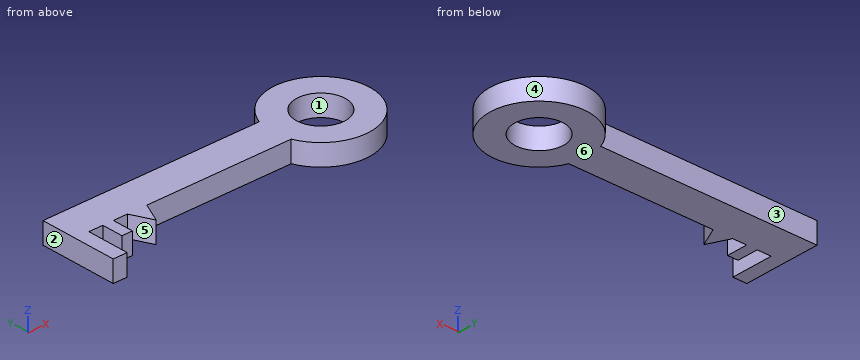
from build123d import *

# Parameters (mm, degrees)
F0_W     = 7.5505197141
F0_H     = 15
F0_W_2   = 10
F0_H_2   = 30
F0_R     = 17.5
F1_DEPTH = 15


# Not quite as in the source:
# - a feature of the source that left no trace in its solid (it failed there, or was rolled back) is left out


with BuildPart() as f1:
    # F0 (on Top) → F1 (new body)
    with BuildSketch(Plane.XY):
        Polygon((63.855322471, 51.9168977576), (-91.144677529, 51.9168977576), (-91.144677529, 26.9168977576), (-81.144677529, 26.9168977576), (-71.144677529, 26.9168977576), (-63.594157815, 26.9168977576), (-53.594157815, 26.9168977576), (-46.594157815, 26.9168977576), (-39.594157815, 26.9168977576), (63.855322471, 26.9168977576), align=None)
        Polygon((-46.594157815, 11.9168977576), (-39.594157815, 26.9168977576), (-46.594157815, 26.9168977576), (-53.594157815, 26.9168977576), align=None)
        with Locations((-67.369417672, 19.4168977576)):
            Rectangle(F0_W, F0_H)
        with Locations((-86.144677529, 11.9168977576)):
            Rectangle(F0_W_2, F0_H_2)
        with BuildLine():
            ThreePointArc((63.855322471, 26.9168977576), (131.5470645475, 39.4168977576), (63.855322471, 51.9168977576))
            Line((63.855322471, 51.9168977576), (63.855322471, 26.9168977576))
        make_face()
        with Locations((96.5470645475, 39.4168977576)):
            Circle(F0_R, mode=Mode.SUBTRACT)
    extrude(amount=F1_DEPTH)


solid = f1.part
Verification items for the finished model (mm, model axes). Face numbers are marked on the shaded views. A direction names the side the tool comes from. Give positions to 0.01 mm unless a question says otherwise; leave off trailing zeros. Order: outer loops, then holes, each group sorted by start corner. A loop starts at its lowest first (then second) coordinate and runs counter-clockwise, first axis right, second up. Notation, with made-up numbers: M 15,31 L 57,31 A28 ccw 57,56 Z; hole C 11.5,80 d10. An arc over 180 degrees is marked long. Use one line per item in the form item = value. Start each with the question number.
Q1. Section check A-A (x = 98.5). Enter the section's corners in (y, z).
Q2. Section check D-D (x = -19). Enter the section's corners in (y, z).
Q3. Go/stop test with flat-tipped pins: pin 1 Ø2 at (x, z) = (22.5, 9.5) entering from +Y; pin 2 Ø5 at (x, z) = (-75.5, 4.5) entering from -Y; pin 3 Ø4.5 at (y, z) = (5, 5) entering from +X. Record where each tip stops, or that it passes through.
Q4. Access from +Z, -Z, +X, -X, +Y, -Y to the whole of each face (thin tool, end or side, straight path). Record for the marked faces 5 and 6.
Q5. Scan lines: line 1 along X through (y, z) = (18, 4.75); line 2 along Y through (x, z) = (-5.5, 6); line 3 along X through (y, z) = (48.5, 4.25). Record each from-to range of solid material in increasing order. Write a range as [from, to].
Q6. Section check B-B (y = 6.5). Enter the section's corners in (x, z).
Q7. Mould release check, pull along Y, two halves, no side actions. Record for the marked faces 1, 2, 3 and 4: +Y half, -Y half, draft (parallel to the pull), parting line (faces both ways), or undercut.
Q8. Section check C-C (z = 5.5). Enter the section's corners in (x, y).
Evaluation:
q1.outline = M 4.47,0 L 22.03,0 L 22.03,15 L 4.47,15 Z; M 56.81,0 L 74.36,0 L 74.36,15 L 56.81,15 Z
q2.outline = M 26.92,0 L 51.92,0 L 51.92,15 L 26.92,15 Z
q3.pin_1 = 51.92
q3.pin_2 = 26.92
q3.pin_3 = 110.34
q4.face_5 = +Z, -Z, -Y
q4.face_6 = -Z, +X, -X, +Y, -Y
q5.line_1 = [-91.14, -81.14], [-71.14, -63.59], [-49.43, -43.76], [68.86, 124.23]
q5.line_2 = [26.92, 51.92]
q5.line_3 = [-91.14, 81.59], [111.51, 130.35]
q6.outline = M -91.14,0 L -81.14,0 L -81.14,15 L -91.14,15 Z; M 84.65,0 L 108.44,0 L 108.44,15 L 84.65,15 Z
q7.face_1 = undercut
q7.face_2 = draft
q7.face_3 = +Y half
q7.face_4 = parting line
q8.outline = M -91.14,-3.08 L -81.14,-3.08 L -81.14,26.92 L -71.14,26.92 L -71.14,11.92 L -63.59,11.92 L -63.59,26.92 L -53.59,26.92 L -46.59,11.92 L -39.59,26.92 L 63.86,26.92 A35 ccw long 63.86,51.92 L -91.14,51.92 Z; hole C 96.55,39.42 d35
